Answer from the drawing. Dimensions are ordinates in mm from the lowest x, y and z of the part. A direction names the side the tool comes from. Give positions to 0.01 mm unless a question says otherwise; leave off trailing zeros. Order: outer loops, then holes, each group sorted by start corner. A loop starts at its lowest first (then second) coordinate and runs counter-clockwise, first axis right, second up. Notation, with made-up numbers: (-15.5, 72) - (8.5, 72) arc R17 ccw to (8.5, 99) - close; hole circle Ø1 at (77, -12). An arc over 180 degrees is marked (long way). Use a Markdown table: item, result. Add a question column.
1) Find section D-D, the plane x = 12.5. Determine the outline of the cut face in (y, z).
2) The mould has two halves that part along Z. Classify the marked faces 3, 4 and 5: released by +Z, released by -Z, zero draft, split by the parting line, or undercut.
3) Straight lines are drawn through the part: line 1 (Z direction, x = 20.5, y = 14); line 2 (X direction, y = 1, z = 16.5); line 3 (Z direction, x = 19.25, y = 12.5). For each, find the intervals that lie inside material, in ascending order.
4) Find section B-B, the plane z = 14.5. Determine the outline of the cut face in (x, y).
5) Find section C-C, the plane y = 13. Determine the outline of the cut face in (x, z).
6) Find section A-A, the plane x = 20.5. Determine the outline of the cut face in (y, z).
7) For the marked faces 1 and 2, determine the directions among +Z, -Z, +X, -X, +Y, -Y from which every point of the face is accessible in a straight line to the end or side of a thin tool.
8) A flat-ended cylindrical pin translates along its axis: pin 1 (5.5 mm diameter, centred on x = 15, y = 12, fed in from +Z). Find the tip coordinate at first contact, or state that the pin passes through.
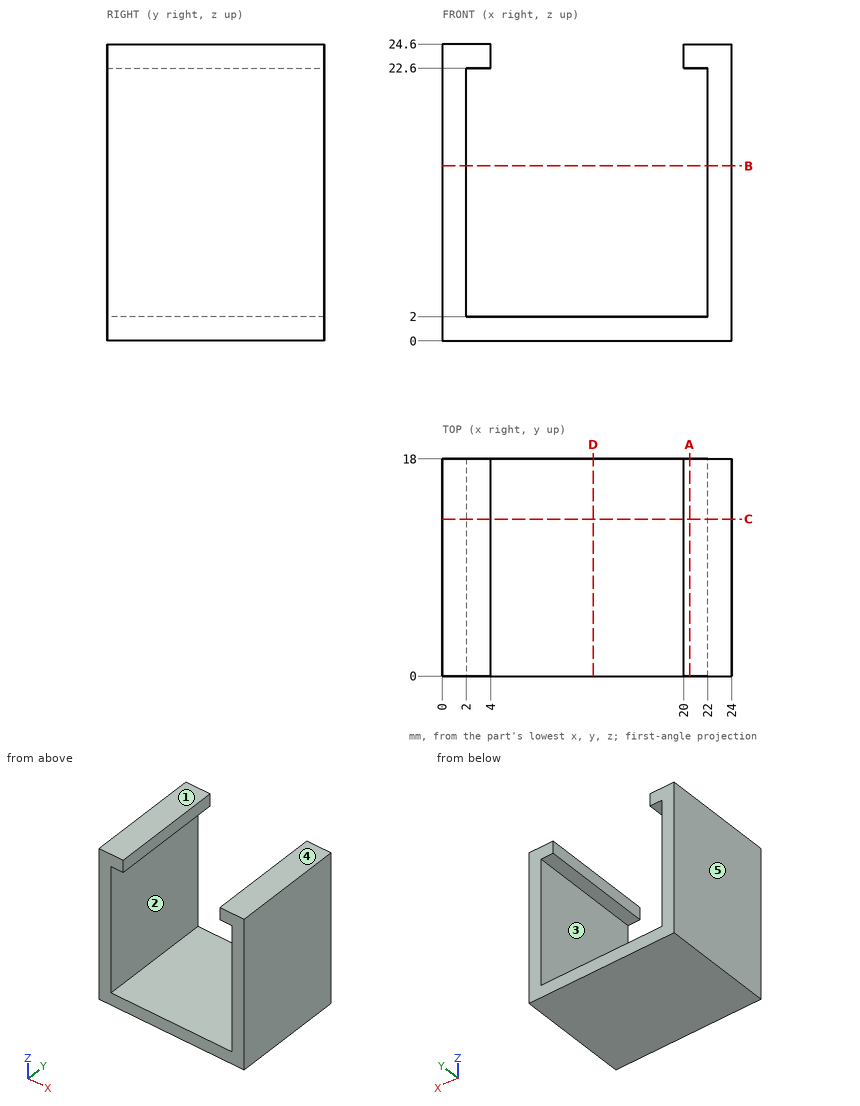
The answers:
| question | item | result |
|---|---|---|
| 1 | outline | (0, 0) - (18, 0) - (18, 2) - (0, 2) - close |
| 2 | face 3 | undercut |
| 2 | face 4 | released by +Z |
| 2 | face 5 | zero draft |
| 3 | line 1 | 0 to 2, 22.6 to 24.6 |
| 3 | line 2 | 0 to 2, 22 to 24 |
| 3 | line 3 | 0 to 2 |
| 4 | outline | (0, 0) - (2, 0) - (2, 18) - (0, 18) - close; (22, 0) - (24, 0) - (24, 18) - (22, 18) - close |
| 5 | outline | (0, 0) - (24, 0) - (24, 24.6) - (20, 24.6) - (20, 22.6) - (22, 22.6) - (22, 2) - (2, 2) - (2, 22.6) - (4, 22.6) - (4, 24.6) - (0, 24.6) - close |
| 6 | outline | (0, 0) - (18, 0) - (18, 2) - (0, 2) - close; (0, 22.6) - (18, 22.6) - (18, 24.6) - (0, 24.6) - close |
| 7 | face 1 | +Z, +X, -X, +Y, -Y |
| 7 | face 2 | +Y, -Y |
| 8 | pin 1 | z = 2 |
